```python
from build123d import *

# Parameters (mm, degrees)
SKETCH_1_W          = 30
SKETCH_1_H          = 30
SKETCH_1_W_2        = 26
SKETCH_1_H_2        = 26
EXTRUDE_1_DEPTH     = 230
SKETCH_2_R          = 2.1
SKETCH_2_R_2        = 2.05
CUT_EXTRUDE_1_DEPTH = 233.432785983
SKETCH_4_R          = 1.55
CUT_EXTRUDE_2_DEPTH = 233.432785983


with BuildPart() as part:
    # 草图1 → 凸台-拉伸1 (new body)
    with BuildSketch(Plane.XY):
        Rectangle(SKETCH_1_W, SKETCH_1_H)
        Rectangle(SKETCH_1_W_2, SKETCH_1_H_2, mode=Mode.SUBTRACT)
    extrude(amount=EXTRUDE_1_DEPTH)

    # 草图2 → 切除-拉伸1 (cut, through all)
    with BuildSketch(Plane.XZ.offset(15)):
        with Locations(Location((-7.5, 10, 0), (0, 0, 270))):
            Circle(SKETCH_2_R)
        with Locations(Location((7.5, 10, 0), (0, 0, 270))):
            Circle(SKETCH_2_R)
        with Locations(Location((7.5, 30, 0), (0, 0, 270))):
            Circle(SKETCH_2_R)
        with Locations(Location((7.5, 50, 0), (0, 0, 270))):
            Circle(SKETCH_2_R)
        with Locations(Location((-7.5, 30, 0), (0, 0, 270))):
            Circle(SKETCH_2_R)
        with Locations(Location((-7.5, 50, 0), (0, 0, 270))):
            Circle(SKETCH_2_R)
        with Locations(Location((-9, 215, 0), (0, 0, 270))):
            Circle(SKETCH_2_R_2)
        with Locations(Location((9, 215, 0), (0, 0, 270))):
            Circle(SKETCH_2_R_2)
        with Locations(Location((9, 190, 0), (0, 0, 270))):
            Circle(SKETCH_2_R_2)
        with Locations(Location((9, 165, 0), (0, 0, 270))):
            Circle(SKETCH_2_R_2)
        with Locations(Location((-9, 190, 0), (0, 0, 270))):
            Circle(SKETCH_2_R_2)
        with Locations(Location((-9, 165, 0), (0, 0, 270))):
            Circle(SKETCH_2_R_2)
    extrude(amount=-CUT_EXTRUDE_1_DEPTH, mode=Mode.SUBTRACT)

    # 草图4 → 切除-拉伸2 (cut, through all)
    with BuildSketch(Plane(origin=(15, 0, 0), x_dir=(0, 0, -1), z_dir=(1, 0, 0))):
        with Locations((-20, 7.5)):
            Circle(SKETCH_4_R)
        with Locations((-40, 7.5)):
            Circle(SKETCH_4_R)
        with Locations((-40, -7.5)):
            Circle(SKETCH_4_R)
        with Locations((-20, -7.5)):
            Circle(SKETCH_4_R)
    extrude(amount=-CUT_EXTRUDE_2_DEPTH, mode=Mode.SUBTRACT)


solid = part.part
```
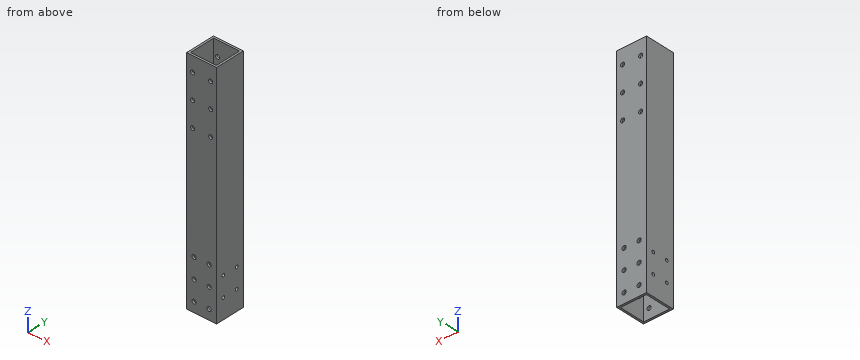
The model under review builds one solid part; all positions refer to its coordinate system, in mm. Round coordinates to 2 decimals unless told otherwise and drop trailing zeros. Write each loop counter-clockwise with the first axis right and the second up, starting at its lowest first coordinate (ties: lowest second). Pieces come first, ordered by that corner, then holes.
(1) We need section D-D on z = 165. Give the boundary of the cut face in (x, y), and give its area (3 significant figures).
(2) Wall thickness on L1, parallel to X at y = -14.2, z = 10; L2, parallel to Y at x = 5.5, z = 195.5; L3, parallel to Y at x = -13.8, z = 20: over which ranges is each line inside the solid? List them lowest first.
(3) We need section B-B on y = 3. Give the boundary of the cut face in (x, z).
(4) We need section A-A on z = 50. Give the boundary of the cut face in (x, y), and give its area (3 significant figures).
Findings below:
1. outline: (-15, -15) - (-11.05, -15) - (-11.05, -13) - (-13, -13) - (-13, 13) - (-11.05, 13) - (-11.05, 15) - (-15, 15) - close; (-6.95, -15) - (6.95, -15) - (6.95, -13) - (-6.95, -13) - close; (-6.95, 13) - (6.95, 13) - (6.95, 15) - (-6.95, 15) - close; (11.05, -15) - (15, -15) - (15, 15) - (11.05, 15) - (11.05, 13) - (13, 13) - (13, -13) - (11.05, -13) - close
1. area: 191 mm2
2. L1: x = -15 to -9.6, -5.4 to 5.4, 9.6 to 15
2. L2: y = -15 to -13, 13 to 15
2. L3: y = -15 to -9.05, -5.95 to 5.95, 9.05 to 15
3. outline: (-15, 0) - (-13, 0) - (-13, 230) - (-15, 230) - close; (13, 0) - (15, 0) - (15, 230) - (13, 230) - close
4. outline: (-15, -15) - (-9.6, -15) - (-9.6, -13) - (-13, -13) - (-13, 13) - (-9.6, 13) - (-9.6, 15) - (-15, 15) - close; (-5.4, -15) - (5.4, -15) - (5.4, -13) - (-5.4, -13) - close; (-5.4, 13) - (5.4, 13) - (5.4, 15) - (-5.4, 15) - close; (9.6, -15) - (15, -15) - (15, 15) - (9.6, 15) - (9.6, 13) - (13, 13) - (13, -13) - (9.6, -13) - close
4. area: 190 mm2
